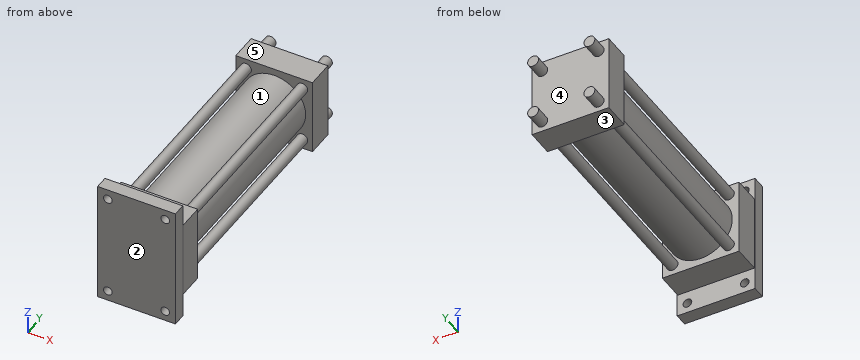
from build123d import *

# Parameters (mm, degrees)
CROQUIS1_W              = 114.3
CROQUIS1_H              = 180
SALIENTE_EXTRUIR1_DEPTH = 19.05
CROQUIS2_R              = 6.35
CORTAR_EXTRUIR1_DEPTH   = 19.05
CROQUIS3_W              = 112.7125
CROQUIS3_H              = 112.7125
SALIENTE_EXTRUIR2_DEPTH = 40
CROQUIS4_R              = 8
CORTAR_EXTRUIR2_DEPTH   = 40
CROQUIS5_R              = 8
SALIENTE_EXTRUIR3_DEPTH = 338
CROQUIS6_R              = 38.1
CORTAR_EXTRUIR3_DEPTH   = 10
CROQUIS7_R              = 46.355
SALIENTE_EXTRUIR4_DEPTH = 298
CROQUIS8_W              = 112.7125
CROQUIS8_H              = 112.7125
SALIENTE_EXTRUIR5_DEPTH = 40
CROQUIS9_R              = 8
SALIENTE_EXTRUIR6_DEPTH = 24


with BuildPart() as part:
    # Croquis1 → Saliente-Extruir1 (new body)
    with BuildSketch(Plane(origin=(0, 0, 0), x_dir=(1, 0, 0), z_dir=(0, 1, 0))):
        Rectangle(CROQUIS1_W, CROQUIS1_H)
    extrude(amount=SALIENTE_EXTRUIR1_DEPTH)

    # Croquis2 → Cortar-Extruir1 (cut)
    with BuildSketch(Plane(origin=(0, 19.05, 0), x_dir=(1, 0, 0), z_dir=(0, 1, 0))):
        with Locations((-42.15, 75)):
            Circle(CROQUIS2_R)
        with Locations((42.15, 75)):
            Circle(CROQUIS2_R)
        with Locations((42.15, -75)):
            Circle(CROQUIS2_R)
        with Locations((-42.15, -75)):
            Circle(CROQUIS2_R)
    extrude(amount=-CORTAR_EXTRUIR1_DEPTH, mode=Mode.SUBTRACT)

    # Croquis3 → Saliente-Extruir2 (add)
    with BuildSketch(Plane(origin=(0, 19.05, 0), x_dir=(1, 0, 0), z_dir=(0, 1, 0))):
        Rectangle(CROQUIS3_W, CROQUIS3_H)
    extrude(amount=SALIENTE_EXTRUIR2_DEPTH)

    # Croquis4 → Cortar-Extruir2 (cut)
    with BuildSketch(Plane(origin=(0, 59.05, 0), x_dir=(1, 0, 0), z_dir=(0, 1, 0))):
        with Locations((-41.35625, 41.35625)):
            Circle(CROQUIS4_R)
        with Locations((41.35625, 41.35625)):
            Circle(CROQUIS4_R)
        with Locations((41.35625, -41.35625)):
            Circle(CROQUIS4_R)
        with Locations((-41.35625, -41.35625)):
            Circle(CROQUIS4_R)
    extrude(amount=-CORTAR_EXTRUIR2_DEPTH, mode=Mode.SUBTRACT)

    # Croquis5 → Saliente-Extruir3 (add)
    with BuildSketch(Plane(origin=(0, 19.05, 0), x_dir=(1, 0, 0), z_dir=(0, 1, 0))):
        with Locations((-41.35625, 41.35625)):
            Circle(CROQUIS5_R)
        with Locations((41.35625, 41.35625)):
            Circle(CROQUIS5_R)
        with Locations((41.35625, -41.35625)):
            Circle(CROQUIS5_R)
        with Locations((-41.35625, -41.35625)):
            Circle(CROQUIS5_R)
    extrude(amount=SALIENTE_EXTRUIR3_DEPTH)

    # Croquis6 → Cortar-Extruir3 (cut)
    with BuildSketch(Plane(origin=(0, 59.05, 0), x_dir=(1, 0, 0), z_dir=(0, 1, 0))):
        Circle(CROQUIS6_R)
    extrude(amount=-CORTAR_EXTRUIR3_DEPTH, mode=Mode.SUBTRACT)

    # Croquis7 → Saliente-Extruir4 (add)
    with BuildSketch(Plane(origin=(0, 59.05, 0), x_dir=(1, 0, 0), z_dir=(0, 1, 0))):
        Circle(CROQUIS7_R)
    extrude(amount=SALIENTE_EXTRUIR4_DEPTH)

    # Croquis8 → Saliente-Extruir5 (add)
    with BuildSketch(Plane(origin=(0, 357.05, 0), x_dir=(1, 0, 0), z_dir=(0, 1, 0))):
        Rectangle(CROQUIS8_W, CROQUIS8_H)
    extrude(amount=SALIENTE_EXTRUIR5_DEPTH)

    # Croquis9 → Saliente-Extruir6 (add)
    with BuildSketch(Plane(origin=(0, 397.05, 0), x_dir=(1, 0, 0), z_dir=(0, 1, 0))):
        with Locations((-41.35625, 41.35625)):
            Circle(CROQUIS9_R)
        with Locations((41.35625, 41.35625)):
            Circle(CROQUIS9_R)
        with Locations((-41.35625, -41.35625)):
            Circle(CROQUIS9_R)
        with Locations((41.35625, -41.35625)):
            Circle(CROQUIS9_R)
    extrude(amount=SALIENTE_EXTRUIR6_DEPTH)


solid = part.part
Geometry: final body of the model. Coordinates: model frame, mm. Face numbers are marked on the shaded views. A direction names the side the tool comes from. Coordinates: 2 decimals unless noted, no trailing zeros. Loops run counter-clockwise (first coordinate to the right, second up) from the corner with the lowest first, then second, coordinate; pieces in that order, holes last. Notation, with made-up numbers: M 83.25,-38 L 117.25,-38 A25 cw 117.25,-23 Z; hole C 79,52.25 d10. An arc over 180 degrees is marked long. One line per item, written item: value. Start each with the question number.
1) Material intervals for L1, parallel to Z at x = -42, y = 11; L2, parallel to X at y = 12, z = -75; L3, parallel to Z at x = -39, y = 351, sorted ascending. Write a range as from..to.
2) Draft query along X for the marked faces 4 and 5. Return one class per face: released by +X, released by -X, zero draft, split by the parting line, or undercut.
3) Cut plane A-A (z = 75). Return loops of the section in (x, y).
4) Pin query (flat end, axial travel): P1, Ø10, axis at x = 42.15, z = -75, coming from the +Y side; P2, Ø20, axis at y = 47.5, z = -11.5, coming from the -X side; P3, Ø12, axis at y = 120.5, z = -29.5, coming from the -X side; P4, Ø20, axis at x = -9.5, y = 35, coming from the +Z side. Return the tip coordinate at first contact, or that it passes through.
5) Reachability of the marked faces 1, 2 and 3 from +Z, -Z, +X, -X, +Y, -Y: full face, straight path, thin tool, end or side. Return the list, or none.
6) Cut plane B-B (x = 0). Return loops of the section in (y, z) (3 decimals).
7) Cut plane C-C (z = 0). Return loops of the section in (x, y) (3 decimals).
8) Cut plane D-D (y = 298). Return loops of the section in (x, z) (3 decimals), then the cut area to 3 significant figures.
Evaluation:
1. L1: -90..-81.35, -68.65..68.65, 81.35..90
1. L2: -57.15..-48.5, -35.8..35.8, 48.5..57.15
1. L3: -49..-33.71, -25.06..25.06, 33.71..49
2. face 4: undercut
2. face 5: zero draft
3. outline: M -57.15,0 L -48.5,0 L -48.5,19.05 L -57.15,19.05 Z; M -35.8,0 L 35.8,0 L 35.8,19.05 L -35.8,19.05 Z; M 48.5,0 L 57.15,0 L 57.15,19.05 L 48.5,19.05 Z
4. P1: through
4. P2: x = -56.36
4. P3: x = -46.81
4. P4: z = 56.36
5. face 1: none
5. face 2: +Z, -Z, +X, -X, -Y
5. face 3: -Z, +X, -X, +Y
6. outline: M 0,-90 L 19.05,-90 L 19.05,-56.356 L 59.05,-56.356 L 59.05,-46.355 L 357.05,-46.355 L 357.05,-56.356 L 397.05,-56.356 L 397.05,56.356 L 357.05,56.356 L 357.05,46.355 L 59.05,46.355 L 59.05,56.356 L 19.05,56.356 L 19.05,90 L 0,90 Z; hole M 49.05,-38.1 L 59.05,-38.1 L 59.05,38.1 L 49.05,38.1 Z
7. outline: M -57.15,0 L 57.15,0 L 57.15,19.05 L 56.356,19.05 L 56.356,59.05 L 46.355,59.05 L 46.355,357.05 L 56.356,357.05 L 56.356,397.05 L -56.356,397.05 L -56.356,357.05 L -46.355,357.05 L -46.355,59.05 L -56.356,59.05 L -56.356,19.05 L -57.15,19.05 Z; hole M -38.1,49.05 L 38.1,49.05 L 38.1,59.05 L -38.1,59.05 Z
8. outline: C -41.356,-41.356 d16; C -41.356,41.356 d16; C 0,0 d92.71; C 41.356,-41.356 d16; C 41.356,41.356 d16
8. area: 7,550 mm^2
